Here's how the part is built. I have some questions about the finished solid (model axes, mm). Face numbers are marked on the shaded views. Give positions to 0.01 mm unless a question says otherwise; leave off trailing zeros. Loops run counter-clockwise (first coordinate to the right, second up) from the corner with the lowest first, then second, coordinate; pieces in that order, holes last.
Q1. Thinking about a two-plate mould opening in X: for the marked faces 1 and 2, which applies, pulls with the +X half, pulls with the -X half, needs draft (parallel to the pull), parting line crosses it, or undercut?
Q2. I'm going to push flat-ended pins straight in: P1, Ø10, axis at x = 1373.5, z = 682, coming from the -Y side; P2, Ø8, axis at y = 285, z = 771.5, coming from the +X side; P3, Ø3, axis at y = 389.5, z = 899.5, coming from the -X side. Where does each tip first touch, or does it pass through?
Q3. I need wall thicknesses on probe 1 along X at (y, z) = (819.5, 349.5); probe 2 along X at (y, z) = (776, 457); probe 3 along Y at (x, z) = (1074.5, 700). Which ranges of each line are inside material? Lowest first, please.
Q4. Suppose I cut it at B-B (z = 603.5). List the corners of the cut face in (x, y) for me, and give its area (3 significant figures).
```python
from build123d import *

# Parameters (mm, degrees)
BOSS_EXTRUDE1_DEPTH = 1018.2
FILLET1_START       = -1
FILLET1_DEPTH       = 10
FILLET1_START_2     = 2027
FILLET1_2_DEPTH     = 11


with BuildPart() as part:
    # Sketch1 → Boss-Extrude1 (new body)
    with BuildSketch(Plane.XY):
        with BuildLine():
            Line((2036.872393674, 565.728630714), (2033.445329339, 563.665809819))
            ThreePointArc((2033.445329339, 563.665809819), (814.110783703, 1055.756928134), (4.181650628, 19.926245878))
            Line((4.181650628, 19.926245878), (0.182315406, 19.99916901))
            ThreePointArc((0.182315406, 19.99916901), (813.075507523, 1059.620631439), (2036.872393674, 565.728630714))
        make_face()
    extrude(amount=BOSS_EXTRUDE1_DEPTH)

    # Fillet1: read off the stored shape, not the designer's step
    # Fillet1 outline → Fillet1 (cut)
    with BuildSketch(Plane(origin=(0, 0, 0), x_dir=(0.018230783053814693, 0.9998338054643106, 0), z_dir=(0.9998338054643106, -0.018230783053814693, 0)).offset(FILLET1_START)):
        with BuildLine():
            ThreePointArc((119.99916901, 0), (49.288490891, 29.289321881), (19.99916901, 100))
            Line((19.99916901, 100), (19.99916901, 0))
            Line((19.99916901, 0), (119.99916901, 0))
        make_face()
        with BuildLine():
            ThreePointArc((19.99916901, 918.2), (49.288490891, 988.910678119), (119.99916901, 1018.2))
            Line((119.99916901, 1018.2), (19.99916901, 1018.2))
            Line((19.99916901, 1018.2), (19.99916901, 918.2))
        make_face()
    extrude(amount=FILLET1_DEPTH, mode=Mode.SUBTRACT)

    # Fillet1 2 outline → Fillet1 2 (cut)
    with BuildSketch(Plane(origin=(0, 0, 0), x_dir=(0.5157052239876767, -0.8567660835676328, 0), z_dir=(0.8567660835676328, 0.515705223987677, 0)).offset(FILLET1_START_2)):
        with BuildLine():
            Line((565.728630715, 0), (465.728630715, 0))
            ThreePointArc((465.728630715, 0), (536.439308834, -29.289321881), (565.728630715, -100))
            Line((565.728630715, -100), (565.728630715, 0))
        make_face()
        with BuildLine():
            Line((565.728630715, -1018.2), (565.728630715, -918.2))
            ThreePointArc((565.728630715, -918.2), (536.439308834, -988.910678119), (465.728630715, -1018.2))
            Line((465.728630715, -1018.2), (565.728630715, -1018.2))
        make_face()
    extrude(amount=FILLET1_2_DEPTH, mode=Mode.SUBTRACT)


solid = part.part
```
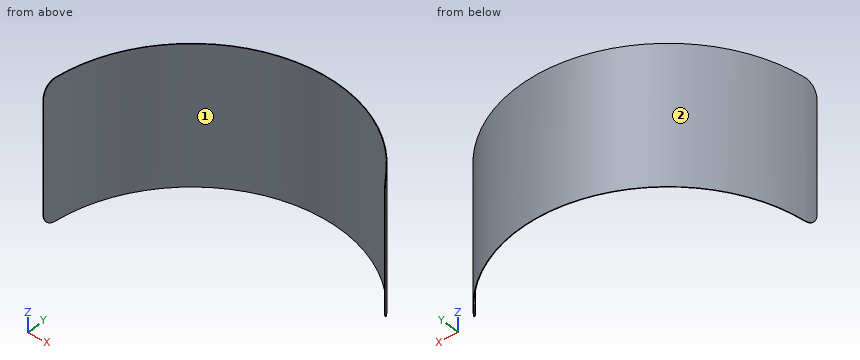
Solutions:
1. face 1: undercut
1. face 2: parting line crosses it
2. P1: stops at y = 1056.13
2. P2: stops at x = 42.9
2. P3: stops at x = 70.91
3. probe 1: x = 367.73 to 373.77, 1820.23 to 1826.27
3. probe 2: x = 321.61 to 327.28, 1866.72 to 1872.39
3. probe 3: y = 1092.77 to 1096.77
4. outline: (0.18, 20) - (4.18, 19.93) arc R1093 cw to (2033.45, 563.67) - (2036.87, 565.73) arc R1097 ccw to start
4. area: 11,300 mm2
